from build123d import *

# Parameters (mm, degrees)
F0_W     = 127
F0_H     = 55.5625
F1_DEPTH = 1117.6
F2_W     = 44.45
F2_H     = 50.8
F3_DEPTH = 55.5635
F5_DEPTH = 1073.151
F6_R     = 55.56249


# Not quite as in the source:
# - a fillet or chamfer is up to 0.001 mm smaller than in the source, because OpenCascade refuses the exact size


with BuildPart() as f1:
    # F0 (on Right) → F1 (new body)
    with BuildSketch(Plane.YZ):
        Rectangle(F0_W, F0_H)
    extrude(amount=F1_DEPTH)

    # F2 (on face) → F3 (cut, through all)
    with BuildSketch(Plane.XY.offset(27.78125)):
        with Locations((22.225, -38.1)):
            Rectangle(F2_W, F2_H)
        with Locations((1095.375, -38.1)):
            Rectangle(F2_W, F2_H)
    extrude(amount=-F3_DEPTH, mode=Mode.SUBTRACT)

    # F4 (on face) → F5 (cut, through all)
    with BuildSketch(Plane.YZ.offset(1073.15)):
        with BuildLine():
            Line((-38.1, 0), (-44.5271766257, -7.0297244343))
            ThreePointArc((-44.5271766257, -7.0297244343), (-38.1, -9.525), (-31.6728233743, -7.0297244343))
            Line((-31.6728233743, -7.0297244343), (-38.1, 0))
        make_face()
        with BuildLine():
            ThreePointArc((-44.5271766257, 7.0297244343), (-47.625, 0), (-44.5271766257, -7.0297244343))
            Line((-44.5271766257, -7.0297244343), (-38.1, 0))
            Line((-38.1, 0), (-44.5271766257, 7.0297244343))
        make_face()
        with BuildLine():
            Line((-44.5271766257, 7.0297244343), (-38.1, 0))
            Line((-38.1, 0), (-31.6728233743, 7.0297244343))
            ThreePointArc((-31.6728233743, 7.0297244343), (-38.1, 9.525), (-44.5271766257, 7.0297244343))
        make_face()
        with BuildLine():
            Line((-31.6728233743, 7.0297244343), (-38.1, 0))
            Line((-38.1, 0), (-31.6728233743, -7.0297244343))
            ThreePointArc((-31.6728233743, -7.0297244343), (-29.3837943359, -3.8410133845), (-28.575, 0))
            ThreePointArc((-28.575, 0), (-29.3837943359, 3.8410133845), (-31.6728233743, 7.0297244343))
        make_face()
    extrude(amount=-F5_DEPTH, mode=Mode.SUBTRACT)

    # F6 (radius 55.5625 in the source; OpenCascade refuses exactly that, so slightly less here)
    f6_edges = [f1.edges().sort_by_distance(p)[0] for p in [
        (558.8, -63.5, -27.78125),
    ]]
    fillet(f6_edges, radius=F6_R)


solid = f1.part
The model under review builds one solid part; all positions refer to its coordinate system, in mm. A direction names the side the tool comes from. Round coordinates to 2 decimals unless told otherwise and drop trailing zeros. Loops run counter-clockwise (first coordinate to the right, second up) from the corner with the lowest first, then second, coordinate; pieces in that order, holes last. Notation, with made-up numbers: (49, -37) - (100, -37) arc R15 ccw to (100, -28) - close; hole circle Ø3 at (55.25, 23.25). An arc over 180 degrees is marked (long way). Use CSV: the item, a comma, the result in double quotes.
(1) For line 1 (X direction, y = -45.5, z = 14); line 2 (Z direction, x = 782, y = -30); line 3 (Y direction, x = 503, z = -4), list the stretches that pass through material, from the lowest coordinate up.
Working result:
line 1,"x = 44.45 to 1073.15"
line 2,"z = -23.21 to -5.01, 5.01 to 27.78"
line 3,"y = -53.51 to -46.74, -29.46 to 63.5"
(2) Clearance check with flat-ended pins moving along their axes: P1, Ø4, axis at x = 949.5, y = -11, coming from the -Z side; P2, Ø15, axis at y = -26, z = -1, coming from the -X side; P3, Ø6, axis at x = 226, z = 18.5, coming from the -Y side. State where each tip first meets the part, or that it passes through.
Working result:
P1,"stops at z = -27.77"
P2,"stops at x = 44.45"
P3,"stops at y = -63.14"
(3) Machinability: for faces 1 (the flat face through (551, 27, -27.781)), 2 (the flat face through (1073.15, -27, 7)), 3 (the flat face through (22, -12.7, 0)), which of the approach directions +Z, -Z, +X, -X, +Y, -Y give a long, thin tool a straight path to every point of the face, cutting with its end or side? Answer none if there is none.
Working result:
face 1,"-Z, +X, -X, +Y, -Y"
face 2,"+Z, -Z, +X, -Y"
face 3,"+Z, -Z, -X, -Y"
(4) Take a section at B-B, the plane z = 18. Give the boundary of the cut face in (x, y), plus the area to 3 significant figures.
Working result:
outline,"(0, -12.7) - (44.45, -12.7) - (44.45, -62.63) - (1073.15, -62.63) - (1073.15, -12.7) - (1117.6, -12.7) - (1117.6, 63.5) - (0, 63.5) - close"
area,"137,000 mm^2"
